Autodesk Inventor part; units mm, degrees
ref_plane "YZ Plane" through (0, 0, 0) normal (1, 0, 0) x (0, 1, 0)
ref_plane "XZ Plane" through (0, 0, 0) normal (0, 1, 0) x (-1, 0, 0)
ref_plane "XY Plane" through (0, 0, 0) normal (0, 0, 1) x (1, 0, 0)
sketch "Sketch1" plane through (0, 0, 0) normal (0, 1, 0) x (-1, 0, 0)
  line L0 (0, 0) -> (25.654, 0)
  line L1 (25.654, 0) -> (25.654, -62.23)
  line L2 (25.654, -62.23) -> (0, -62.23)
  line L3 (0, -62.23) -> (0, 0)
  circle A0 centre (3.302, -3.302) radius 1.27
  circle A1 centre (3.302, -59.182) radius 1.27
  circle A2 centre (22.352, -3.302) radius 1.27
  circle A3 centre (22.352, -59.182) radius 1.27
  dimension "d0" = 25.654
  dimension "d1" = 2.54
  dimension "d2" = 3.302
  dimension "d3" = 3.302
  dimension "d4" = 62.23
  dimension "d7" = 55.88
  dimension "d10" = 19.05
extrude "Extrusion1" add sketch "Sketch1" along normal blind 1.524
sketch "Sketch2" plane through (0, 1.524, 0) normal (0, 1, 0) x (1, 0, 0)
  circle A0 centre (-19.177, 2.032) radius 0.51
  line L0 (-25.654, 0) -> (0, 0)
  circle A1 centre (-16.637, 2.032) radius 0.51
  circle A2 centre (-14.097, 2.032) radius 0.51
  circle A3 centre (-11.557, 2.032) radius 0.51
  circle A4 centre (-9.017, 2.032) radius 0.51
  circle A5 centre (-6.477, 2.032) radius 0.51
  circle A6 centre (-22.352, 3.302) radius 1.27
  circle A7 centre (-6.604, 7.112) radius 0.51
  line L1 (-25.654, 62.23) -> (-25.654, 0)
  circle A8 centre (-6.604, 9.652) radius 0.51
  circle A9 centre (-6.604, 12.192) radius 0.51
  circle A10 centre (-6.604, 14.732) radius 0.51
  circle A11 centre (-4.064, 7.112) radius 0.51
  circle A12 centre (-4.064, 9.652) radius 0.51
  circle A13 centre (-4.064, 12.192) radius 0.51
  circle A14 centre (-4.064, 14.732) radius 0.51
  circle A15 centre (-1.524, 7.112) radius 0.51
  circle A16 centre (-1.524, 9.652) radius 0.51
  circle A17 centre (-1.524, 12.192) radius 0.51
  circle A18 centre (-1.524, 14.732) radius 0.51
  circle A19 centre (-3.302, 3.302) radius 1.27
  line L2 (0, 0) -> (0, 62.23)
  circle A20 centre (-4.064, 19.812) radius 0.51
  circle A21 centre (-1.524, 19.812) radius 0.51
  circle A22 centre (-1.524, 22.352) radius 0.51
  circle A23 centre (-6.604, 24.892) radius 0.51
  circle A24 centre (-4.064, 24.892) radius 0.51
  circle A25 centre (-1.524, 24.892) radius 0.51
  circle A26 centre (-6.604, 27.432) radius 0.51
  circle A27 centre (-4.064, 27.432) radius 0.51
  circle A28 centre (-1.524, 27.432) radius 0.51
  circle A29 centre (-6.604, 22.352) radius 0.51
  circle A30 centre (-4.064, 22.352) radius 0.51
  circle A31 centre (-6.604, 19.812) radius 0.51
  circle A32 centre (-1.524, 37.592) radius 0.51
  circle A33 centre (-4.064, 37.592) radius 0.51
  circle A34 centre (-6.604, 37.592) radius 0.51
  circle A35 centre (-1.524, 40.132) radius 0.51
  circle A36 centre (-4.064, 40.132) radius 0.51
  circle A37 centre (-6.604, 40.132) radius 0.51
  circle A38 centre (-1.524, 42.672) radius 0.51
  circle A39 centre (-4.064, 42.672) radius 0.51
  circle A40 centre (-6.604, 42.672) radius 0.51
  circle A41 centre (-4.064, 35.052) radius 0.51
  circle A42 centre (-1.524, 35.052) radius 0.51
  circle A43 centre (-6.604, 35.052) radius 0.51
  circle A44 centre (-4.064, 47.752) radius 0.51
  circle A45 centre (-1.524, 47.752) radius 0.51
  circle A46 centre (-6.604, 47.752) radius 0.51
  circle A47 centre (-4.064, 50.292) radius 0.51
  circle A48 centre (-6.604, 50.292) radius 0.51
  circle A49 centre (-1.524, 50.292) radius 0.51
  circle A50 centre (-4.064, 52.832) radius 0.51
  circle A51 centre (-6.604, 52.832) radius 0.51
  circle A52 centre (-1.524, 52.832) radius 0.51
  circle A53 centre (-6.604, 55.372) radius 0.51
  circle A54 centre (-4.064, 55.372) radius 0.51
  circle A55 centre (-1.524, 55.372) radius 0.51
  circle A56 centre (-6.477, 60.198) radius 0.51
  circle A57 centre (-9.017, 60.198) radius 0.51
  circle A58 centre (-11.557, 60.198) radius 0.51
  circle A59 centre (-19.177, 60.198) radius 0.51
  circle A60 centre (-16.637, 60.198) radius 0.51
  circle A61 centre (-14.097, 60.198) radius 0.51
  dimension "d15" = 1.02
  dimension "d16" = 2.032
  dimension "d19" = 2.54
  dimension "d24" = 3.175
  dimension "d25" = 1.02
  dimension "d28" = 2.54
  dimension "d31" = 2.54
  dimension "d34" = 4.064
  dimension "d35" = 9.652
  dimension "d38" = 12.7
  dimension "d45" = 15.24
  dimension "d52" = 12.7
  dimension "d63" = 58.166
extrude "Extrusion4" cut sketch "Sketch2" against normal through all contours A0 | A1 | A2 | A3 | A4 | A5 | A7 | A8 | A9 | A10 | A11 | A12 | A13 | A14 | A15 | A16 | A17 | A18 | A20 | A21 | A22 | A23 | A24 | A25 | A26 | A27 | A28 | A29 | A30 | A31 | A32 | A33 | A34 | A35 | A36 | A37 | A38 | A39 | A40 | A41 | A42 | A43 | A44 | A45 | A46 | A47 | A48 | A49 | A50 | A51 | A52 | A53 | A54 | A55 | A56 | A57 | A58 | A59 | A60 | A61
fillet "Fillet1" radius 3.302 4 edges at (-25.654, 0.762, 0) (0, 0.762, 0) (0, 0.762, -62.23) (-25.654, 0.762, -62.23)
properties part number "MainPCB" material "Silicon Nitride"
For this review, take the finished solid that the model builds, in its own axes (mm). Give positions to 0.01 mm unless a question says otherwise; leave off trailing zeros. Loops run counter-clockwise (first coordinate to the right, second up) from the corner with the lowest first, then second, coordinate; pieces in that order, holes last. Notation, with made-up numbers: M 9.25,46.25 L 13.25,46.25 A31 ccw 13.25,83.25 Z; hole C 7,43.25 d8. An arc over 180 degrees is marked long. One line per item, written item: value. Start each with the question number.
Q1. For L1, parallel to X at y = 0.55, z = -7; L2, parallel to Z at x = -11.25, y = 0.1; L3, parallel to X at y = 1.3, z = -19.5, list the stretches that pass through material, from the lowest coordinate up.
Q2. Clearance check with a flat-ended pin moving along its axis: pin 1 Ø1.2 at (x, z) = (-11.557, -60.198) entering from -Y. State where the tip first meets the part, or that it passes through.
Q3. Add section B-B (y = 0.75). Count the separate pieces of the cut face and the enclosed holes in it, and give its area (3 significant figures).
Q4. Draft analysis for pull direction Z (two halves, no side actions). For faces 1 (the face through (-11.67, 0.77, -59.7)), 2 (the face through (-24.66, 0.77, -61.29)), 3 (the face through (-25.654, 1, -31)), state which applies: released by +Z, released by -Z, zero draft, split by the parting line, or undercut.
Q5. Add section A-A (x = -23). Give the boundary of the cut face in (y, z), and give its area (3 significant figures).
Reply:
1. L1: -25.65 to -7.1, -6.11 to -4.56, -3.57 to -2.02, -1.03 to 0
1. L2: -62.23 to -60.61, -59.79 to -2.44, -1.62 to 0
1. L3: -25.65 to -7.01, -6.2 to -4.47, -3.66 to -1.93, -1.12 to 0
2. pin 1: y = 0
3. separate pieces: 1
3. enclosed holes: 64
3. area: 1,520 mm²
4. face 1: undercut
4. face 2: released by -Z
4. face 3: zero draft
5. outline: M 0,-62.17 L 1.52,-62.17 L 1.52,-60.27 L 0,-60.27 Z; M 0,-58.09 L 1.52,-58.09 L 1.52,-4.39 L 0,-4.39 Z; M 0,-2.21 L 1.52,-2.21 L 1.52,-0.06 L 0,-0.06 Z
5. area: 88.0 mm²
